```python
from build123d import *

# Parameters (mm, degrees)
BOSS_EXTRUDE1_DEPTH = 20
SKETCH6_R           = 1.6
CUT_EXTRUDE4_DEPTH  = 16.556349186
SKETCH7_R           = 2.7
CUT_EXTRUDE5_DEPTH  = 10.556349186
FILLET4_R           = 1
FILLET5_R           = 0.5
CUT_EXTRUDE6_DEPTH  = 10
CUT_EXTRUDE7_DEPTH  = 10
FILLET6_R           = 1.5


with BuildPart() as part:
    # Sketch1 → Boss-Extrude1 (new body)
    with BuildSketch(Plane.XY):
        Polygon((0, 0), (0, 15.556349186), (15.556349186, 0), align=None)
    extrude(amount=BOSS_EXTRUDE1_DEPTH)

    # Sketch6 → Cut-Extrude4 (cut, through all)
    with BuildSketch(Plane.ZY):
        with Locations((16.335044769, 3.811593223)):
            Circle(SKETCH6_R)
        with Locations((3.664955231, 3.811593223)):
            Circle(SKETCH6_R)
    extrude(amount=-CUT_EXTRUDE4_DEPTH, mode=Mode.SUBTRACT)

    # Sketch7 → Cut-Extrude5 (cut, through all)
    with BuildSketch(Plane.ZY.offset(-6)):
        with Locations((16.335044769, 3.811593223)):
            Circle(SKETCH7_R)
        with Locations((3.664955231, 3.811593223)):
            Circle(SKETCH7_R)
    extrude(amount=-CUT_EXTRUDE5_DEPTH, mode=Mode.SUBTRACT)

    # Fillet4
    fillet4_edges = [part.edges().sort_by_distance(p)[0] for p in [
        (0, 0, 10),
    ]]
    fillet(fillet4_edges, radius=FILLET4_R)

    # Fillet5
    fillet5_edges = [part.edges().sort_by_distance(p)[0] for p in [
        (0, 15.556349186, 10),
        (15.556349186, 0, 10),
    ]]
    fillet(fillet5_edges, radius=FILLET5_R)

    # Sketch8 → Cut-Extrude6 (cut)
    with BuildSketch(Plane(origin=(7.778174593, 7.778174593, 0), x_dir=(0, 0, -1), z_dir=(0.707106781, 0.707106781, 0))):
        Polygon((-20, -12.333051339), (0, -12.333051339), (0.012190886, -3.93058749), (-20, -3.93058749), align=None)
    extrude(amount=-CUT_EXTRUDE6_DEPTH, mode=Mode.SUBTRACT)

    # Sketch9 → Cut-Extrude7 (cut)
    with BuildSketch(Plane(origin=(7.778174593, 7.778174593, 0), x_dir=(0, 0, -1), z_dir=(0.707106781, 0.707106781, 0))):
        Polygon((-11.323221056, 10.808771842), (0, 5.528667149), (0, 10.808771842), align=None)
    extrude(amount=-CUT_EXTRUDE7_DEPTH, mode=Mode.SUBTRACT)

    # Fillet6
    fillet6_edges = [part.edges().sort_by_distance(p)[0] for p in [
        (8.058104899, 2.499414762, 0),
        (1.934408281, 9.753124344, 0),
    ]]
    fillet(fillet6_edges, radius=FILLET6_R)


solid = part.part
```
Read the model definition and answer for the solid it produces. Units are mm, in the model's axes. A direction names the side the tool comes from. Coordinates: 2 decimals unless noted, no trailing zeros. Loops run counter-clockwise (first coordinate to the right, second up) from the corner with the lowest first, then second, coordinate; pieces in that order, holes last. Notation, with made-up numbers: (-10, 62) -> (33, 62) arc R28 cw to (33, 97) -> close; hole circle Ø8 at (50, -3). An arc over 180 degrees is marked (long way). Return JSON: item names as keys, results as strings.
Item 1: Find section D-D (x = 1.5). Count the separate pieces of the cut face and the enclosed holes in it, plus the area to 3 significant figures.
Answers:
{"separate pieces": "1", "enclosed holes": "2", "area": "248 mm2"}
Item 2: Find section C-C (y = 12.5). Determine the outline of the cut face in (x, z).
Answers:
{"outline": "(0, 7.1) -> (3.06, 2.46) -> (3.06, 20) -> (0, 20) -> close"}
Item 3: Find section A-A (z = 4). Determine the outline of the cut face in (x, y), plus the area to 3 significant figures.
Answers:
{"outline": "(0, 1) arc R1 ccw to (1, 0) -> (5.56, 0) -> (6.69, 1.13) -> (6, 1.13) -> (6, 2.25) -> (0, 2.25) -> close; (0, 5.38) -> (6, 5.38) -> (6, 6.49) -> (9.07, 6.49) -> (2.55, 13.01) -> (0, 10.46) -> close", "area": "54.7 mm2"}
Item 4: Flat-ended cylindrical pins translate along their axes: P1, Ø2, axis at x = 7, z = 11.5, coming from the -Y side; P2, Ø1.5, axis at y = 3, z = 12, coming from the -X side; P3, Ø3, axis at y = 6.5, z = 3, coming from the +X side; P4, Ø4, axis at y = 11, z = 11, coming from the +X side. Find the tip coordinate at first contact, or state that the pin passes through.
Answers:
{"P1": "stops at y = 0.44", "P2": "stops at x = 0", "P3": "stops at x = 9.86", "P4": "stops at x = 6.56"}
Item 5: Find the intervals of material crossed by probe 1 along Z at (x, y) = (8, 4.5); probe 2 along Y at (x, z) = (2, 3); probe 3 along X at (y, z) = (3, 14), in increasing order.
Answers:
{"probe 1": "z = 0 to 1.05, 6.28 to 13.72, 18.95 to 20", "probe 2": "y = 0 to 2.36, 5.27 to 11.8", "probe 3": "x = 0 to 6"}
Item 6: For faces 1 (the cylindrical face through (0.285, 0.301, 10.14)), 2 (the flat face through (6, 2, 16)), determine the directions among +Z, -Z, +X, -X, +Y, -Y from which every point of the face is accessible in a straight line to the end or side of a thin tool.
Answers:
{"face 1": "+Z, -Z, -X, -Y", "face 2": "+X"}
Item 7: For a pull along Y with two mould halves and no side action, classify faces 3 (the cylindrical face through (2.18, 9.78, 0.23)), 4 (the flat face through (3, 0, 10)), 5 (the cylindrical face through (7.74, 6.49, 3.31)) as +Y half, -Y half, draft (parallel to the pull), parting line (faces both ways), or undercut.
Answers:
{"face 3": "+Y half", "face 4": "-Y half", "face 5": "undercut"}
Item 8: Find section B-B (z = 12.25). Determine the outline of the cut face in (x, y), plus the area to 3 significant figures.
Answers:
{"outline": "(0, 1) arc R1 ccw to (1, 0) -> (5.56, 0) -> (10.56, 5) -> (0.85, 14.7) arc R0.5 ccw to (0, 14.35) -> close", "area": "95.5 mm2"}
